from build123d import *

# Parameters (mm, degrees)
SKETCH1_R               = 12.5
BOSS_EXTRUDE1_DEPTH     = 5
BOSS_EXTRUDE2_DEPTH     = 2
CUT_EXTRUDE1_DEPTH      = 19.371173071
CUT_EXTRUDE1_DEPTH_BACK = 19.371173071
SKETCH7_R               = 1.5


with BuildPart() as part:
    # Sketch1 → Boss-Extrude1 (new body)
    with BuildSketch(Plane(origin=(0, 0, 0), x_dir=(1, 0, 0), z_dir=(0, 1, 0))):
        with Locations(Location((0, 0, 0), (0, 0, 270))):
            Circle(SKETCH1_R)
    extrude(amount=BOSS_EXTRUDE1_DEPTH)

    # Sketch5 → Boss-Extrude2 (add)
    with BuildSketch(Plane.XZ):
        with BuildLine():
            ThreePointArc((0.151933345, 9.240024976), (7.241529429, -4.84837498), (-7.728040184, 0.117243971))
            ThreePointArc((-7.728040184, 0.117243971), (4.587114181, -2.555573928), (0.151933345, 9.240024976))
        make_face()
        with BuildLine():
            ThreePointArc((-3.656517397, -6.557691991), (-5.001923128, -5.543170647), (-6.121751206, -4.284061751))
            Line((-6.121751206, -4.284061751), (-6.613956363, -5.53781326))
            Line((-6.613956363, -5.53781326), (-9.1213874, -7.458398735))
            Line((-9.1213874, -7.458398735), (-9.1213874, -7.938927068))
            Line((-9.1213874, -7.938927068), (-3.783058525, -7.938927068))
            Line((-3.783058525, -7.938927068), (-3.783058525, -7.698853884))
            Line((-3.783058525, -7.698853884), (-3.656517397, -6.557691991))
        make_face()
        with BuildLine():
            ThreePointArc((6.332224885, -5.753540044), (5.494878341, -6.385314366), (4.586346954, -6.909584092))
            Line((4.586346954, -6.909584092), (4.398231289, -7.803613119))
            Line((4.398231289, -7.803613119), (8.835264261, -7.803613119))
            Line((8.835264261, -7.803613119), (8.835264261, -7.356598606))
            Line((8.835264261, -7.356598606), (6.332224885, -5.753540044))
        make_face()
        with BuildLine():
            ThreePointArc((-0.950626232, 8.887896426), (2.400955984, -1.341013908), (-7.728040184, 2.301395544))
            ThreePointArc((-7.728040184, 2.301395544), (2.870290324, -1.823952142), (-0.950626232, 8.887896426))
        make_face()
        with BuildLine():
            ThreePointArc((-5.206948691, -1.953864639), (-4.267011364, -2.491822801), (-3.245572389, -2.851744431))
            Line((-3.245572389, -2.851744431), (-3.200349413, -2.443918626))
            Line((-3.200349413, -2.443918626), (0.032158273, 5.78996786))
            Line((0.032158273, 5.78996786), (2.539505861, -1.201879249))
            ThreePointArc((2.539505861, -1.201879249), (3.172462056, -0.424101438), (3.666799623, 0.448367609))
            Line((3.666799623, 0.448367609), (0.151933345, 8.626753393))
            ThreePointArc((0.151933345, 8.626753393), (-0.393157926, 8.783453154), (-0.950626232, 8.887896426))
            Line((-0.950626232, 8.887896426), (-5.206948691, -1.953864639))
        make_face()
        with BuildLine():
            ThreePointArc((1.577176372, 0.117243971), (0.166068053, -1.570987631), (-1.245040266, 0.117243971))
            Line((-1.245040266, 0.117243971), (0.032158273, 3.12312116))
            Line((0.032158273, 3.12312116), (1.577176372, 0.117243971))
        make_face()
    extrude(amount=BOSS_EXTRUDE2_DEPTH)

    # Sketch7 → Cut-Extrude1 (cut, two sides: drawn at the far end of the back side and taken through both)
    with BuildSketch(Plane.XZ.offset(-CUT_EXTRUDE1_DEPTH_BACK)):
        with Locations(Location((-7.119157088, 7.022649241, 0), (0, 0, 270))):
            Circle(SKETCH7_R)
    extrude(amount=CUT_EXTRUDE1_DEPTH + CUT_EXTRUDE1_DEPTH_BACK, mode=Mode.SUBTRACT)


solid = part.part
Can you work these out from the model? Positions are in its coordinate system, mm. A direction names the side the tool comes from. Coordinates: 2 decimals unless noted, no trailing zeros. Loops run counter-clockwise (first coordinate to the right, second up) from the corner with the lowest first, then second, coordinate; pieces in that order, holes last. Notation, with made-up numbers: M 14.25,-8.5 L 45.25,-8.5 A22 cw 45.25,8.5 Z; hole C 39.5,57 d4. An arc over 180 degrees is marked long. Return JSON: item names as keys, results as strings. Group by question number.
Item 1: Imagine slicing it at D-D (x = -9.5). Please give me the cut outline in (y, z).
Item 2: Thinking about a two-plate mould opening in Z: for faces 5 (the flat face through (2.9, -2, -4.4)), 6 (the flat face through (0.794, -0.986, 1.641)), 7 (the flat face through (-3.72, -0.99, -7.14)), which applies, released by +Z, released by -Z, zero draft, split by the parting line, or undercut?
Item 3: I'm going to push flat-ended pins straight in: pin 1 Ø1 at (x, y) = (-5.5, 1.5) entering from -Z; pin 2 Ø3 at (y, z) = (3, 5) entering from -X; pin 3 Ø3.5 at (x, z) = (-7.12, 7.02) entering from -Y; pin 4 Ø4 at (x, z) = (-3.5, -3.5) entering from -Y. Where does each tip first touch, or does it pass through?
Item 4: Imagine slicing it at A-A (z = 3.75). Please give me the cut outline in (x, y), and give its area (3 significant figures).
Item 5: If I drill on L1, parallel to X at y = -1, z = 6.5; L2, parallel to Y at x = -0.5, z = -8.75; L3, parallel to X at y = 4.5, z = 6, over which ranges is the centre line in solid material (lowest first)? Write a range as from..to.
Item 6: Imagine slicing it at C-C (y = 4). Please give me the cut outline in (x, z), and give its area (3 significant figures).
Item 7: On a 3-axis mill with a long thin cutter (end or side, diameter ignored), from which of +Z, -Z, +X, -X, +Y, -Y can I reach the whole of each face in a straight line? I mean faces 1 (the flat face through (-7.85, -0.986, -6.485)), 2 (the cylindrical face through (2.725, -0.986, -1.961)), 3 (the flat face through (-6, -1, -7.939)), 4 (the flat face through (7.601, -0.986, -6.566)). Say none if no direction works.
Item 8: Imagine slicing it at B-B (x = -1.75). Please give me the cut outline in (y, z), and give its area (3 significant figures).
Verdict:
{
 "1": {"outline": "M 0,-8.12 L 5,-8.12 L 5,8.12 L 0,8.12 Z"},
 "2": {"face 5": "zero draft", "face 6": "undercut", "face 7": "released by -Z"},
 "3": {"pin 1": "stops at z = -11.46", "pin 2": "stops at x = -12", "pin 3": "stops at y = 0", "pin 4": "stops at y = -2"},
 "4": {"outline": "M -11.92,0 L -2.97,0 L -2.97,-2 L -0.77,-2 L -0.77,0 L 0.76,0 L 0.76,-2 L 2.25,-2 L 2.25,0 L 4.16,0 L 4.16,-2 L 4.67,-2 L 4.67,0 L 6.15,0 L 6.15,-2 L 8.76,-2 L 8.76,0 L 11.92,0 L 11.92,5 L -11.92,5 Z", "area": "133 mm^2"},
 "5": {"L1": "x = -1.89..1.07, 3.05..3.45, 4.85..7.07", "L2": "y = 0..5", "L3": "x = -10.97..-8.22, -6.02..10.97"},
 "6": {"outline": "C 0,0 d25; hole C -7.12,7.02 d3", "area": "484 mm^2"},
 "7": {"face 1": "-X, -Y", "face 2": "-Y", "face 3": "-Z, +X, -X, -Y", "face 4": "+X, -Y"},
 "8": {"outline": "M -2,-7.42 L 0,-7.42 L 0,-12.38 L 5,-12.38 L 5,12.38 L 0,12.38 L 0,6.85 L -2,6.85 L -2,1.25 L 0,1.25 L 0,-3.04 L -2,-3.04 L -2,-3.59 L 0,-3.59 L 0,-4.98 L -2,-4.98 Z", "area": "141 mm^2"}
}
